from build123d import *

# Parameters (mm, degrees)
SKETCH001_R      = 1.5
EXTRUDE001_DEPTH = 10
EXTRUDE_DEPTH    = 5


with BuildPart() as extrude001:
    # Sketch001 (on Face6 of Extrude) → Extrude001 (new body, symmetric)
    with BuildSketch(Plane.YZ.offset(1.5)):
        with Locations((-4.883141, 2.5)):
            Circle(SKETCH001_R)
    extrude(amount=EXTRUDE001_DEPTH, both=True)


with BuildPart() as cut:
    # Sketch → Extrude (new body)
    with BuildSketch(Plane.XY):
        with BuildLine():
            ThreePointArc((0.5, -2.193741), (0, 2.25), (-0.5, -2.193741))
            Line((-0.5, -2.193741), (-0.5, -6.883141))
            Line((-0.5, -6.883141), (-1.5, -6.883141))
            Line((-1.5, -6.883141), (-1.5, -2.883141))
            ThreePointArc((1.5, -2.883141), (0, 3.25), (-1.5, -2.883141))
            Line((1.5, -6.883141), (1.5, -2.883141))
            Line((0.5, -6.883141), (1.5, -6.883141))
            Line((0.5, -2.193741), (0.5, -6.883141))
        make_face()
    extrude(amount=EXTRUDE_DEPTH)

    # Cut: cut Extrude001
    add(extrude001.part, mode=Mode.SUBTRACT)


solid = cut.part
The listing builds one solid part. Answer for the finished solid, in the listing's coordinates (mm). A direction names the side the tool comes from. Round coordinates to 2 decimals unless told otherwise and drop trailing zeros. Loops run counter-clockwise (first coordinate to the right, second up) from the corner with the lowest first, then second, coordinate; pieces in that order, holes last. Notation, with made-up numbers: M 29.25,79 L 81.25,79 A7 cw 81.25,84 Z; hole C -36,86.25 d3. An arc over 180 degrees is marked long. Write each question's results on one line, items separated by ' | '. Start each with the question number.
1) Find section B-B on y = 0. Write down the section's boundary in (x, z).
2) Find section A-A on z = 2.5. Write down the section's boundary in (x, y).
3) Find section C-C on x = 1. Write down the section's boundary in (y, z).
4) Each of these flat-tipped pins is pushed along its axis until it touches: pin 1 (1 mm diameter, centred on x = 1, y = 0, fed in from -Z); pin 2 (1 mm diameter, centred on x = 1, z = 2.5, fed in from +Y); pin 3 (2.5 mm diameter, centred on y = -5.5, z = 2, fed in from -X); pin 4 (2 mm diameter, centred on y = -5, z = 3.5, fed in from +X). Where does it stop, or does it pass through?
5) Which of the six approach directions +Z, -Z, +X, -X, +Y, -Y give full straight-line access (tool end or side, diameter ignored) to faces 1 (the flat face through (-1.5, -4.9, 0.8)), 2 (the flat face through (1.5, -4.9, 0.8)), 3 (the flat face through (1, -3, 0)), 4 (the flat face through (0.5, -3, 2))?
6) Straight lines are drawn through the part: probe 1 along Y at (x, z) = (-1, 3.8); probe 2 along Y at (x, z) = (-1, 1.75); probe 3 along X at (y, z) = (0, 4.1). For each, find the intervals that lie inside material, in ascending order.
7) Determine the mould class of faces 5 (the cylindrical face through (1.01, -4.19, 1.17)), 6 (the flat face through (1, -3, 5)), 7 (the cylindrical face through (-0.99, -4.19, 1.17)), 8 (the flat face through (-0.5, -3, 2)) for opening direction Z: pulls with the +Z half, pulls with the -Z half, needs draft (parallel to the pull), parting line crosses it, or undercut.
8) Find section D-D on z = 4.55. Write down the section's boundary in (x, y).
Final values:
1) outline: M -3.25,0 L -2.25,0 L -2.25,5 L -3.25,5 Z; M 2.25,0 L 3.25,0 L 3.25,5 L 2.25,5 Z
2) outline: M -1.5,-6.88 L -0.5,-6.88 L -0.5,-6.38 L -1.5,-6.38 Z; M -1.5,-3.38 L -0.5,-3.38 L -0.5,-2.19 A2.25 cw long 0.5,-2.19 L 0.5,-3.38 L 1.5,-3.38 L 1.5,-2.88 A3.25 ccw long -1.5,-2.88 Z; M 0.5,-6.88 L 1.5,-6.88 L 1.5,-6.38 L 0.5,-6.38 Z
3) outline: M -6.88,0 L -2.02,0 L -2.02,5 L -6.88,5 Z; M 2.02,0 L 3.09,0 L 3.09,5 L 2.02,5 Z; hole C -4.88,2.5 d3
4) pin 1: through | pin 2: y = 3.21 | pin 3: x = -1.5 | pin 4: x = 1.5
5) face 1: +Z, -Z, -X, -Y | face 2: +Z, -Z, +X, -Y | face 3: -Z, +X, -X, +Y, -Y | face 4: +Z, -Z, -Y
6) probe 1: -6.88 to -5.63, -4.13 to -2.02, 2.02 to 3.09 | probe 2: -6.88 to -6.18, -3.58 to -2.02, 2.02 to 3.09 | probe 3: -3.25 to -2.25, 2.25 to 3.25
7) face 5: undercut | face 6: pulls with the +Z half | face 7: undercut | face 8: needs draft
8) outline: M -1.5,-6.88 L -0.5,-6.88 L -0.5,-2.19 A2.25 cw long 0.5,-2.19 L 0.5,-6.88 L 1.5,-6.88 L 1.5,-2.88 A3.25 ccw long -1.5,-2.88 Z
